For this review, take the finished solid that the model builds, in its own axes (mm). A direction names the side the tool comes from. Coordinates: 2 decimals unless noted, no trailing zeros. Order: outer loops, then holes, each group sorted by start corner. A loop starts at its lowest first (then second) coordinate and runs counter-clockwise, first axis right, second up. Notation, with made-up numbers: (-34.5, 9.25) -> (18.5, 9.25) arc R26 cw to (18.5, 37.25) -> close; hole circle Ø11 at (26, -13.75). An arc over 180 degrees is marked (long way). Answer as a JSON object with one key per item and string values. Group by question number.
1) For pin 1 (0.6 mm diameter, centred on y = 3, z = 1.5, fed in from +X); pin 2 (8.5 mm diameter, centred on x = -10, z = 2.5, fed in from +Y); pin 3 (2 mm diameter, centred on x = -12.5, z = 6, fed in from -Y), all flat-tipped, find the tip position at first contact; note any pin that passes through.
2) Wall thickness on L1, parallel to Z at x = -6.25, y = 5.25; L2, parallel to X at y = 5.2, z = -5.75; L3, parallel to Y at x = -7.5, z = -10.25: over which ranges is each line inside the solid? List them lowest first.
3) Add section B-B, the plane y = 3. Count the separate pieces of the cut face and the enclosed holes in it, then the cut area to 3 significant figures.
4) Machinability: for faces 1 (the flat face through (-12, 2.615, 0)), 2 (the flat face through (-7, 3, 4.229)), 3 (the flat face through (-17.628, 3, 0)), which of the approach directions +Z, -Z, +X, -X, +Y, -Y give a long, thin tool a straight path to every point of the face, cutting with its end or side? Answer none if there is none.
5) Draft analysis for pull direction Z (two halves, no side actions). For faces 4 (the cylindrical face through (-5.865, 4.058, -8.405)), 5 (the flat face through (-8.3, 3.7, 12.7)), 6 (the cylindrical face through (-12.85, 3.26, -9.5)), 7 (the flat face through (-4, 6, 4.233)), state which applies: +Z half, -Z half, draft (parallel to the pull), parting line (faces both ways), or undercut.
6) Add section C-C, the plane x = -13. Write out the cut boundary in (y, z), then the cut area to 3 significant figures.
7) Add section D-D, the plane y = 6.8. Write out the cut boundary in (x, z).
8) Add section A-A, the plane z = 6.5. Write out the cut boundary in (x, y), then the cut area to 3 significant figures.
from build123d import *

# Parameters (mm, degrees)
SKETCH2_R                = 1.1811
BOSS_EXTRUDE1_DEPTH      = 12.7
BOSS_EXTRUDE1_DEPTH_BACK = 12.7
SKETCH3_R                = 2.4638
CUT_EXTRUDE1_DEPTH       = 4.23291
CUT_EXTRUDE1_DEPTH_BACK  = 4.2291
SKETCH4_W                = 2.905794066
SKETCH4_H                = 2.259273031
CUT_EXTRUDE2_DEPTH       = 4.2291
CUT_EXTRUDE2_DEPTH_BACK  = 4.2291
FILLET2_R                = 0.254
FILLET3_R                = 0.254
SKETCH5_R                = 1.6637
CUT_EXTRUDE3_DEPTH       = 2.54


with BuildPart() as part:
    # Sketch2 → Boss-Extrude1 (new body, two sides)
    with BuildSketch(Plane.XY) as boss_extrude1_sk:
        with BuildLine():
            Line((-17.6276, 2.614576368), (-17.6276, 3.884576368))
            Line((-17.6276, 3.884576368), (-7.224163794, 3.884576368))
            ThreePointArc((-7.224163794, 3.884576368), (-3.076448638, 6.402723098), (-6.1087, 2.614576368))
            Line((-6.1087, 2.614576368), (-17.6276, 2.614576368))
        make_face()
        with Locations((-4.9276, 4.776823632)):
            Circle(SKETCH2_R, mode=Mode.SUBTRACT)
    extrude(amount=BOSS_EXTRUDE1_DEPTH)
    extrude(boss_extrude1_sk.sketch, amount=-BOSS_EXTRUDE1_DEPTH_BACK)

    # Sketch3 → Cut-Extrude1 (cut, two sides)
    with BuildSketch(Plane.XY) as cut_extrude1_sk:
        with Locations((-4.9276, 4.776823632)):
            Circle(SKETCH3_R)
    extrude(amount=CUT_EXTRUDE1_DEPTH, mode=Mode.SUBTRACT)
    extrude(cut_extrude1_sk.sketch, amount=-CUT_EXTRUDE1_DEPTH_BACK, mode=Mode.SUBTRACT)

    # Sketch4 → Cut-Extrude2 (cut, two sides)
    with BuildSketch(Plane.XY) as cut_extrude2_sk:
        with Locations((-6.438882967, 3.744212884)):
            Rectangle(SKETCH4_W, SKETCH4_H)
    extrude(amount=CUT_EXTRUDE2_DEPTH, mode=Mode.SUBTRACT)
    extrude(cut_extrude2_sk.sketch, amount=-CUT_EXTRUDE2_DEPTH_BACK, mode=Mode.SUBTRACT)

    # Fillet2
    fillet2_edges = [part.edges().sort_by_distance(p)[0] for p in [
        (-7.89178, 3.249576368, -4.2291),
    ]]
    fillet(fillet2_edges, radius=FILLET2_R)

    # Fillet3
    fillet3_edges = [part.edges().sort_by_distance(p)[0] for p in [
        (-7.89178, 3.249576368, 4.2291),
    ]]
    fillet(fillet3_edges, radius=FILLET3_R)

    # Sketch5 → Cut-Extrude3 (cut)
    with BuildSketch(Plane(origin=(0, 3.884576368, 0), x_dir=(1, 0, 0), z_dir=(0, 1, 0))):
        with Locations((-12.6365, 7.8486)):
            Circle(SKETCH5_R)
        with Locations((-12.6365, -7.8486)):
            Circle(SKETCH5_R)
    extrude(amount=-CUT_EXTRUDE3_DEPTH, mode=Mode.SUBTRACT)


solid = part.part
Output values:
{
 "1": {"pin 1": "stops at x = -7.89", "pin 2": "stops at y = 6.93", "pin 3": "stops at y = 2.61"},
 "2": {"L1": "z = -12.7 to -4.23, 4.23 to 12.7", "L2": "x = -7.35 to -6.03, -3.82 to -2.5", "L3": "y = 2.61 to 3.88"},
 "3": {"separate pieces": "1", "enclosed holes": "2", "area": "309 mm²"},
 "4": {"face 1": "+Z, -Z, -X, -Y", "face 2": "+X, +Y, -Y", "face 3": "+Z, -Z, -X, +Y, -Y"},
 "5": {"face 4": "draft", "face 5": "+Z half", "face 6": "undercut", "face 7": "undercut"},
 "6": {"outline": "(2.61, -12.7) -> (3.88, -12.7) -> (3.88, -9.47) -> (2.61, -9.47) -> close; (2.61, -6.23) -> (3.88, -6.23) -> (3.88, 6.23) -> (2.61, 6.23) -> close; (2.61, 9.47) -> (3.88, 9.47) -> (3.88, 12.7) -> (2.61, 12.7) -> close", "area": "24.0 mm²"},
 "7": {"outline": "(-6.33, -12.7) -> (-3.52, -12.7) -> (-3.52, -4.23) -> (-6.33, -4.23) -> close; (-6.33, 4.23) -> (-3.52, 4.23) -> (-3.52, 12.7) -> (-6.33, 12.7) -> close"},
 "8": {"outline": "(-17.63, 2.61) -> (-13.61, 2.61) -> (-13.61, 3.88) -> (-17.63, 3.88) -> close; (-11.66, 2.61) -> (-6.11, 2.61) arc R2.46 ccw (long way) to (-7.22, 3.88) -> (-11.66, 3.88) -> close; hole circle Ø2.36 at (-4.93, 4.78)", "area": "26.0 mm²"}
}
